For this review, take the finished solid that the model builds, in its own axes (mm). A direction names the side the tool comes from. Coordinates: 2 decimals unless noted, no trailing zeros. Order: outer loops, then holes, each group sorted by start corner. A loop starts at its lowest first (then second) coordinate and runs counter-clockwise, first axis right, second up. Notation, with made-up numbers: M 83,88 L 105,88 A14 ccw 105,92 Z; hole C 29,41.25 d6. An arc over 180 degrees is marked long. Use CSV: the item, a comma, the result in double quotes.
```python
from build123d import *

# Parameters (mm, degrees)
F0_W        = 2159
F0_H        = 1600.2
F0_W_2      = 1854.2
F0_H_2      = 1295.4
F1_DEPTH    = 177.8
F2_W        = 76.2
F2_H        = 76.2
F3_DEPTH    = 736.6
F4_T1_DEPTH = 177.8
F4_T3_DEPTH = 812.8
F5_W        = 101.6
F5_H        = 177.8
F6_DEPTH    = 1295.4


# Not quite as in the source:
# - a fillet or chamfer that OpenCascade refuses, or shapes differently, is made with other operations: its cross-section is extruded or revolved along the edge and cut away or added


with BuildPart() as f1:
    # F0 (on Top) → F1 (new body)
    with BuildSketch(Plane.XY):
        with Locations((1079.5, 800.1)):
            Rectangle(F0_W, F0_H)
        with Locations((1079.5, 800.1)):
            Rectangle(F0_W_2, F0_H_2, mode=Mode.SUBTRACT)
    extrude(amount=F1_DEPTH)

    # F2 (on face) → F3 (join)
    with BuildSketch(Plane(origin=(0, 0, 0), x_dir=(1, 0, 0), z_dir=(0, 0, -1))):
        with Locations((114.3, -114.3)):
            Rectangle(F2_W, F2_H)
        with Locations((2044.7, -114.3)):
            Rectangle(F2_W, F2_H)
        with Locations((2044.7, -1485.9)):
            Rectangle(F2_W, F2_H)
        with Locations((114.3, -1485.9)):
            Rectangle(F2_W, F2_H)
    extrude(amount=F3_DEPTH)

    # F4: fillet of radius 127 on 8 edges, made by hand

    # F4_s2 → F4_t1 (join)
    with BuildSketch(Plane.XY):
        with BuildLine():
            ThreePointArc((279.4, 1447.8), (189.5974387893, 1410.6025612107), (152.4, 1320.8))
            Line((152.4, 1320.8), (152.4, 1447.8))
            Line((152.4, 1447.8), (279.4, 1447.8))
        make_face()
        with BuildLine():
            ThreePointArc((2006.6, 1320.8), (1969.4025612107, 1410.6025612107), (1879.6, 1447.8))
            Line((1879.6, 1447.8), (2006.6, 1447.8))
            Line((2006.6, 1447.8), (2006.6, 1320.8))
        make_face()
        with BuildLine():
            ThreePointArc((2006.6, 279.4), (1969.4025612107, 189.5974387893), (1879.6, 152.4))
            Line((1879.6, 152.4), (2006.6, 152.4))
            Line((2006.6, 152.4), (2006.6, 279.4))
        make_face()
        with BuildLine():
            ThreePointArc((152.4, 279.4), (189.5974387893, 189.5974387893), (279.4, 152.4))
            Line((279.4, 152.4), (152.4, 152.4))
            Line((152.4, 152.4), (152.4, 279.4))
        make_face()
    extrude(amount=F4_T1_DEPTH)

    # F4_s4 → F4_t3 (cut)
    with BuildSketch(Plane.XY.offset(-317.5)):
        with BuildLine():
            ThreePointArc((0, 127), (37.1974387893, 37.1974387893), (127, 0))
            Line((127, 0), (0, 0))
            Line((0, 0), (0, 127))
        make_face()
        with BuildLine():
            ThreePointArc((0, 1473.2), (37.1974387893, 1563.0025612107), (127, 1600.2))
            Line((127, 1600.2), (0, 1600.2))
            Line((0, 1600.2), (0, 1473.2))
        make_face()
        with BuildLine():
            ThreePointArc((2032, 0), (2121.8025612107, 37.1974387893), (2159, 127))
            Line((2159, 127), (2159, 0))
            Line((2159, 0), (2032, 0))
        make_face()
        with BuildLine():
            ThreePointArc((2032, 1600.2), (2121.8025612107, 1563.0025612107), (2159, 1473.2))
            Line((2159, 1473.2), (2159, 1600.2))
            Line((2159, 1600.2), (2032, 1600.2))
        make_face()
    extrude(amount=F4_T3_DEPTH, mode=Mode.SUBTRACT)

    # F5 (on face) → F6 (join, through all)
    with BuildSketch(Plane(origin=(0, 152.4, 0), x_dir=(-1, 0, 0), z_dir=(0, 1, 0))):
        with Locations((-1079.5, 88.9)):
            Rectangle(F5_W, F5_H)
    extrude(amount=F6_DEPTH)


solid = f1.part
```
Item 1: For faces 4 (the face through (114, 76.2, -363)), 5 (the face through (114, 1447.8, -363)), 6 (the face through (76.2, 115, -363)), 7 (the face through (2006.6, 115, -363)), 8 (the face through (649, 152.4, 88)), list the 3-axis set-ups (+Z, -Z, +X, -X, +Y, -Y) from which the entire face can be reached by the end or side of a thin tool; tool diameter is ignored.
Solutions:
face 4,"-Z, +X, -X, -Y"
face 5,"-Z, +X, -X"
face 6,"-Z, -X, +Y, -Y"
face 7,"-Z, +Y, -Y"
face 8,"+Z, -Z"
Item 2: To check wall thickness, follow line 1 along Y through (x, z) = (1624.5, 72.5); line 2 along Y through (x, z) = (89, -606.5); line 3 along X through (y, z) = (1482, -653). State the ranges of each line that lie inside material, in increasing order. Write a range as [from, to].
Solutions:
line 1,"[0, 152.4], [1447.8, 1600.2]"
line 2,"[76.2, 152.4], [1447.8, 1524]"
line 3,"[76.2, 152.4], [2006.6, 2082.8]"
Item 3: Draft analysis for pull direction X (two halves, no side actions). For faces 1 (the face through (2044, 1447.8, -363)), 2 (the face through (1500, 1447.8, 88)), 3 (the face through (76.2, 1486, -363)), state which applies: released by +X, released by -X, zero draft, split by the parting line, or undercut.
Solutions:
face 1,"zero draft"
face 2,"undercut"
face 3,"released by -X"
Item 4: Add section D-D on x = 1954. State the section outline as (y, z) points, and give its area (3 significant figures).
Solutions:
outline,"M 0,0 L 176.47,0 L 176.47,177.8 L 0,177.8 Z; M 1423.73,0 L 1600.2,0 L 1600.2,177.8 L 1423.73,177.8 Z"
area,"62,800 mm^2"
Item 5: Add section C-C on x = 1176. State the section outline as (y, z) points, and give its area (3 significant figures).
Solutions:
outline,"M 0,0 L 152.4,0 L 152.4,177.8 L 0,177.8 Z; M 1447.8,0 L 1600.2,0 L 1600.2,177.8 L 1447.8,177.8 Z"
area,"54,200 mm^2"
Item 6: Add section A-A on y = 1244. State the section outline as (x, z) points.
Solutions:
outline,"M 0,0 L 152.4,0 L 152.4,177.8 L 0,177.8 Z; M 1028.7,0 L 1130.3,0 L 1130.3,177.8 L 1028.7,177.8 Z; M 2006.6,0 L 2159,0 L 2159,177.8 L 2006.6,177.8 Z"
Item 7: Clearance check with a flat-ended pin moving along its axis: pin 1 Ø23 at (x, z) = (2048, -389) entering from -Y. State where the tip first meets the part, or that it passes through.
Solutions:
pin 1,"y = 76.2"
Item 8: Add section B-B on z = -141.5. State the section outline as (x, y) points.
Solutions:
outline,"M 76.2,76.2 L 152.4,76.2 L 152.4,152.4 L 76.2,152.4 Z; M 76.2,1447.8 L 152.4,1447.8 L 152.4,1524 L 76.2,1524 Z; M 2006.6,76.2 L 2082.8,76.2 L 2082.8,152.4 L 2006.6,152.4 Z; M 2006.6,1447.8 L 2082.8,1447.8 L 2082.8,1524 L 2006.6,1524 Z"
